from build123d import *

# Parameters (mm, degrees)
SKETCH1_W           = 100
SKETCH1_H           = 100
SKETCH1_R           = 3
BOSS_EXTRUDE1_DEPTH = 10
SKETCH2_R           = 40
BOSS_EXTRUDE2_DEPTH = 40
FILLET1_R           = 5


with BuildPart() as part:
    # Sketch1 → Boss-Extrude1 (new body)
    with BuildSketch(Plane.XY):
        Rectangle(SKETCH1_W, SKETCH1_H)
        with Locations((40, 40)):
            Circle(SKETCH1_R, mode=Mode.SUBTRACT)
        with Locations(Location((-40, 40, 0), (0, 0, 180))):
            Circle(SKETCH1_R, mode=Mode.SUBTRACT)
        with Locations((-40, -40)):
            Circle(SKETCH1_R, mode=Mode.SUBTRACT)
        with Locations(Location((40, -40, 0), (0, 0, 180))):
            Circle(SKETCH1_R, mode=Mode.SUBTRACT)
    extrude(amount=BOSS_EXTRUDE1_DEPTH)

    # Sketch2 → Boss-Extrude2 (add)
    with BuildSketch(Plane.XY.offset(10)):
        Circle(SKETCH2_R)
    extrude(amount=BOSS_EXTRUDE2_DEPTH)

    # Fillet1
    fillet1_edges = [part.edges().sort_by_distance(p)[0] for p in [
        (-40, 0, 50),
        (50, -50, 5),
        (-50, -50, 5),
        (-50, 50, 5),
        (50, 50, 5),
    ]]
    fillet(fillet1_edges, radius=FILLET1_R)


solid = part.part
Geometry: final body of the model. Coordinates: model frame, mm. A direction names the side the tool comes from. Give positions to 0.01 mm unless a question says otherwise; leave off trailing zeros. Loops run counter-clockwise (first coordinate to the right, second up) from the corner with the lowest first, then second, coordinate; pieces in that order, holes last. Notation, with made-up numbers: (10, 42.5) -> (35, 42.5) arc R22 ccw to (35, 70.5) -> close; hole circle Ø6 at (-7.5, 9.5). An arc over 180 degrees is marked (long way). Put each result on its own line as item: value.
1. Cut plane B-B (z = 35.5). Return the cut outline in (x, y), plus the area to 3 significant figures.
Taken from the geometry:
outline: circle Ø80 at (0, 0)
area: 5,030 mm2
2. Cut plane A-A (y = 41.5). Return the cut outline in (x, z), plus the area to 3 significant figures.
Taken from the geometry:
outline: (-50, 0) -> (-42.6, 0) -> (-42.6, 10) -> (-50, 10) -> close; (-37.4, 0) -> (37.4, 0) -> (37.4, 10) -> (-37.4, 10) -> close; (42.6, 0) -> (50, 0) -> (50, 10) -> (42.6, 10) -> close
area: 896 mm2
3. Set-up query: faces 1 (the cylindrical face through (-8.67, -39.05, 27.26)), 2 (the cylindrical face through (48, 49, 5)). Return all of +Z, -Z, +X, -X, +Y, -Y with unobstructed straight access to the full face (end or side cutting, diameter ignored); none if empty.
Taken from the geometry:
face 1: +Z
face 2: +Z, -Z, +X, +Y
4. Pin query (flat end, axial travel): P1, Ø9.5, axis at x = 40, y = -40, coming from the -Z side; P2, Ø5, axis at x = 40, y = 40, coming from the +Z side; P3, Ø5, axis at y = -26, z = 39, coming from the -X side; P4, Ø7, axis at x = -40, y = -40, coming from the +Z side. Return the tip coordinate at first contact, or that it passes through.
Taken from the geometry:
P1: stops at z = 0
P2: passes through
P3: stops at x = -32.37
P4: stops at z = 10
5. Pull-direction query (X, two-part tool) for faces 3 (the flat face through (-34, 23, 10)), 4 (the cylindrical face through (-42.21, -37.97, 4.93)), 5 (the cylindrical face through (-49, 48, 5)); classes: released by +X, released by -X, zero draft, split by the parting line, or undercut.
Taken from the geometry:
face 3: zero draft
face 4: undercut
face 5: released by -X
6. Ray query, line 1 along Y through (x, z) = (40, 6); line 2 along Z through (x, y) = (31.5, 27); line 3 along Y through (x, z) = (-3, 44). Return the intervals inside material, ascending. Write a range as [from, to].
Taken from the geometry:
line 1: y = [-50, -43], [-37, 37], [43, 50]
line 2: z = [0, 10]
line 3: y = [-39.89, 39.89]
